```python
from build123d import *

# Parameters (mm, degrees)
SKETCH2_W           = 150
SKETCH2_H           = 150
BOSS_EXTRUDE1_DEPTH = 20
SKETCH4_W           = 80
SKETCH4_H           = 80
BOSS_EXTRUDE2_DEPTH = 40
SKETCH5_W           = 150
SKETCH5_H           = 150
BOSS_EXTRUDE3_DEPTH = 30
SKETCH6_R           = 13
CUT_EXTRUDE1_DEPTH  = 168
SKETCH7_R           = 21
CUT_EXTRUDE2_DEPTH  = 6
SKETCH8_R           = 32
CUT_EXTRUDE3_DEPTH  = 12
SKETCH9_R           = 7
CUT_EXTRUDE4_DEPTH  = 52


with BuildPart() as part:
    # Sketch2 → Boss-Extrude1 (new body)
    with BuildSketch(Plane(origin=(0, 0, 0), x_dir=(1, 0, 0), z_dir=(0, 1, 0))):
        with Locations((75, 75)):
            Rectangle(SKETCH2_W, SKETCH2_H)
    extrude(amount=BOSS_EXTRUDE1_DEPTH)

    # Sketch4 → Boss-Extrude2 (add)
    with BuildSketch(Plane(origin=(0, 20, 0), x_dir=(1, 0, 0), z_dir=(0, 1, 0))):
        with Locations((75, 75)):
            Rectangle(SKETCH4_W, SKETCH4_H)
    extrude(amount=BOSS_EXTRUDE2_DEPTH)

    # Sketch5 → Boss-Extrude3 (add)
    with BuildSketch(Plane(origin=(0, 60, 0), x_dir=(1, 0, 0), z_dir=(0, 1, 0))):
        with Locations((75, 75)):
            Rectangle(SKETCH5_W, SKETCH5_H)
    extrude(amount=BOSS_EXTRUDE3_DEPTH)

    # Sketch6 → Cut-Extrude1 (cut)
    with BuildSketch(Plane(origin=(0, 90, 0), x_dir=(1, 0, 0), z_dir=(0, 1, 0))):
        with Locations((75, 75)):
            Circle(SKETCH6_R)
    extrude(amount=-CUT_EXTRUDE1_DEPTH, mode=Mode.SUBTRACT)

    # Sketch7 → Cut-Extrude2 (cut)
    with BuildSketch(Plane(origin=(0, 90, 0), x_dir=(1, 0, 0), z_dir=(0, 1, 0))):
        with Locations((75, 75)):
            Circle(SKETCH7_R)
    extrude(amount=-CUT_EXTRUDE2_DEPTH, mode=Mode.SUBTRACT)

    # Sketch8 → Cut-Extrude3 (cut)
    with BuildSketch(Plane.XZ):
        with Locations((75, -75)):
            Circle(SKETCH8_R)
    extrude(amount=-CUT_EXTRUDE3_DEPTH, mode=Mode.SUBTRACT)

    # Sketch9 → Cut-Extrude4 (cut)
    with BuildSketch(Plane(origin=(0, 90, 0), x_dir=(1, 0, 0), z_dir=(0, 1, 0))):
        with Locations((75, 135)):
            Circle(SKETCH9_R)
        with Locations((15, 75)):
            Circle(SKETCH9_R)
        with Locations((75, 15)):
            Circle(SKETCH9_R)
        with Locations((135, 75)):
            Circle(SKETCH9_R)
        with Locations((15, 135)):
            Circle(SKETCH9_R)
        with Locations((135, 135)):
            Circle(SKETCH9_R)
        with Locations((135, 15)):
            Circle(SKETCH9_R)
        with Locations((15, 15)):
            Circle(SKETCH9_R)
    extrude(amount=-CUT_EXTRUDE4_DEPTH, mode=Mode.SUBTRACT)


solid = part.part
```
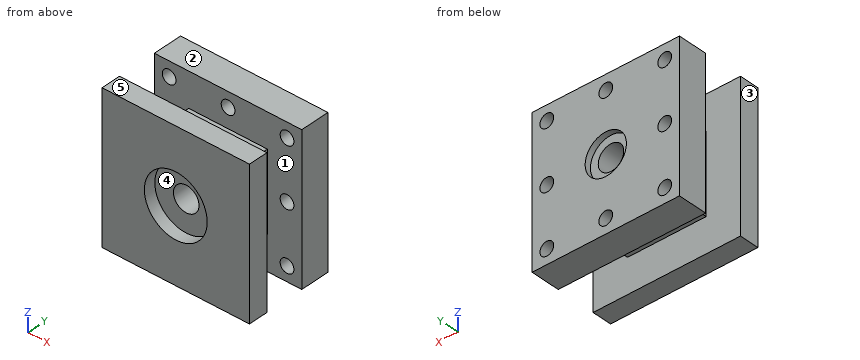
Work out the finished part from the listing and answer in its coordinate system (mm). Face numbers are marked on the shaded views. A direction names the side the tool comes from. Round coordinates to 2 decimals unless told otherwise and drop trailing zeros. Loops run counter-clockwise (first coordinate to the right, second up) from the corner with the lowest first, then second, coordinate; pieces in that order, holes last.
(1) For the marked faces 1 and 2, determine the directions among +Z, -Z, +X, -X, +Y, -Y from which every point of the face is accessible in a straight line to the end or side of a thin tool.
Computed values:
face 1: none
face 2: +Z, +X, -X, +Y, -Y
(2) The mould has two halves that part along X. Classify the marked faces 3, 4 and 5: pulls with the +X half, pulls with the -X half, needs draft (parallel to the pull), parting line crosses it, or undercut.
Computed values:
face 3: pulls with the -X half
face 4: undercut
face 5: needs draft
(3) The part is cut by section D-D, the plane x = 15. Give the vertices of the cut face in (y, z), and give its area (3 significant figures).
Computed values:
outline: (0, -150) - (20, -150) - (20, 0) - (0, 0) - close; (60, -150) - (90, -150) - (90, -142) - (60, -142) - close; (60, -128) - (90, -128) - (90, -82) - (60, -82) - close; (60, -68) - (90, -68) - (90, -22) - (60, -22) - close; (60, -8) - (90, -8) - (90, 0) - (60, 0) - close
area: 6,240 mm2
(4) Each of these flat-tipped pins is pushed along its axis until it touches: P1, Ø4, axis at x = 62, y = 35, coming from the -Z side; P2, Ø12.5, axis at x = 15, z = -75, coming from the +Y side; P3, Ø12, axis at x = 88.5, y = 40, coming from the +Z side. Where does it stop, or does it pass through?
Computed values:
P1: stops at z = -115
P2: stops at y = 20
P3: stops at z = -35
(5) Find the intervals of material crossed by L1, parallel to X at y = 82.5, z = -75; L2, parallel to X at y = 73.75, z = -15; L3, parallel to Z at x = 15, y = 66, in increasing order.
Computed values:
L1: x = 0 to 8, 22 to 62, 88 to 128, 142 to 150
L2: x = 0 to 8, 22 to 68, 82 to 128, 142 to 150
L3: z = -150 to -142, -128 to -82, -68 to -22, -8 to 0
(6) The part is cut by section A-A, the plane x = 75. Give the number of separate pieces and of enclosed holes in the cut face, and give its area (3 significant figures).
Computed values:
separate pieces: 4
enclosed holes: 0
area: 6,970 mm2
(7) The part is cut by section C-C, the plane z = -31. Give the vertices of the cut face in (x, y), and give its area (3 significant figures).
Computed values:
outline: (0, 0) - (150, 0) - (150, 20) - (0, 20) - close; (0, 60) - (150, 60) - (150, 90) - (0, 90) - close
area: 7,500 mm2
